```python
from build123d import *

# Parameters (mm, degrees)
SKETCH_1_W                = 80
SKETCH_1_H                = 51
EXTRUDE_1_DEPTH           = 100
SKETCH_2_W                = 30
SKETCH_2_H                = 35
CUT_EXTRUDE_1_DEPTH       = 131.576605868
SKETCH_3_W                = 54
SKETCH_3_H                = 35
CUT_EXTRUDE_2_DEPTH       = 131.576605868
HOLE_WIZARD_1_D           = 9
HOLE_WIZARD_1_CBORE_D     = 15
HOLE_WIZARD_1_CBORE_DEPTH = 9
MM_1_D                    = 6


with BuildPart() as part:
    # 草图1 → 凸台-拉伸1 (new body)
    with BuildSketch(Plane.XY):
        Rectangle(SKETCH_1_W, SKETCH_1_H)
    extrude(amount=EXTRUDE_1_DEPTH)

    # 草图2 → 切除-拉伸1 (cut, through all)
    with BuildSketch(Plane(origin=(40, 0, 0), x_dir=(0, 0, -1), z_dir=(1, 0, 0))):
        with Locations((-85, -8)):
            Rectangle(SKETCH_2_W, SKETCH_2_H)
    extrude(amount=-CUT_EXTRUDE_1_DEPTH, mode=Mode.SUBTRACT)

    # 草图3 → 切除-拉伸2 (cut, through all)
    with BuildSketch(Plane(origin=(40, 0, 0), x_dir=(0, 0, -1), z_dir=(1, 0, 0))):
        with Locations((-27, 8)):
            Rectangle(SKETCH_3_W, SKETCH_3_H)
    extrude(amount=-CUT_EXTRUDE_2_DEPTH, mode=Mode.SUBTRACT)

    # 打孔尺寸(%根据)内六角圆柱头螺钉的类型1 (through all)
    with Locations(Plane(origin=(0, -9.5, 0), x_dir=(1, 0, 0), z_dir=(0, 1, 0))):
        with Locations((-30, -10), (30, -40)):
            CounterBoreHole(HOLE_WIZARD_1_D / 2, HOLE_WIZARD_1_CBORE_D / 2, HOLE_WIZARD_1_CBORE_DEPTH)

    # 大小mm 暗销孔1 (through all)
    with Locations(Plane(origin=(0, -9.5, 0), x_dir=(1, 0, 0), z_dir=(0, 1, 0))):
        with Locations((-30, -40), (30, -10)):
            Hole(MM_1_D / 2)


solid = part.part
```
Model file for the job. Use its own axes, mm. A direction names the side the tool comes from. Coordinates: 2 decimals unless noted, no trailing zeros. Order: outer loops, then holes, each group sorted by start corner. A loop starts at its lowest first (then second) coordinate and runs counter-clockwise, first axis right, second up. Notation, with made-up numbers: (27, -5.5) - (75, -5.5) arc R16 cw to (75, 24.5) - close; hole circle Ø11 at (47.5, 86). An arc over 180 degrees is marked (long way). Return JSON: item names as keys, results as strings. Group by question number.
1) Flat gauge pins, fed straight in: P1, Ø17.5, axis at x = -17, y = -5, coming from the +Z side; P2, Ø16, axis at x = -18, z = 31, coming from the +Y side; P3, Ø7.5, axis at x = 33.5, z = 39, coming from the +Y side. Where does each tip first touch, or does it go through?
2) Saw through at B-B, the plane z = 40. Write the cut outline in (x, y), plus the area to 3 significant figures.
3) Saw through at C-C, the plane y = -13.5. Write the cut outline in (x, z).
4) Mould opens along X. For faces 6 (the cylindrical face through (-34.292, -22.049, 8.648)), 7 (the flat face through (1, 8, 54)), 8 (the flat face through (-40, -12, 49)), 9 (the cylindrical face through (-27.79, -17.61, 37.97)) say: released by +X, released by -X, zero draft, split by the parting line, or undercut.
5) Saw through at A-A, the plane x = -30. Write the cut outline in (y, z), plus the area to 3 significant figures.
6) Tool access for faces 1 (the cylindrical face through (33, -18, 10)), 2 (the flat face through (-1, -17, 0)), 3 (the flat face through (1, -8, 70)), 4 (the flat face through (1, -9.5, 27)), 5 (the cylindrical face through (-37.493, -13.937, 9.67)): list every direction of +Z, -Z, +X, -X, +Y, -Y with a clear straight run to the whole face (end or side of a thin tool).
7) Probe line 1 (Z direction, x = 30, y = -24); line 2 (Z direction, x = -30, y = -23); line 3 (X direction, y = -11.5, z = 40). List the from-to ranges inside material, lowest first. Write a range as from..to.
8) Saw through at D-D, the plane x = 20.5. Write the cut outline in (y, z).
Values found:
{
 "1": {"P1": "stops at z = 70", "P2": "stops at y = -9.5", "P3": "stops at y = -18.5"},
 "2": {"outline": "(-40, -25.5) - (-33, -25.5) - (-33, -9.5) - (-40, -9.5) - close; (-27, -25.5) - (25.5, -25.5) - (25.5, -18.5) - (22.5, -18.5) - (22.5, -9.5) - (-27, -9.5) - close; (34.5, -25.5) - (40, -25.5) - (40, -9.5) - (37.5, -9.5) - (37.5, -18.5) - (34.5, -18.5) - close", "area": "986 mm²"},
 "3": {"outline": "(-40, 0) - (40, 0) - (40, 70) - (-40, 70) - close; hole circle Ø15 at (-30, 10); hole circle Ø6 at (-30, 40); hole circle Ø15 at (30, 40); hole circle Ø6 at (30, 10)"},
 "4": {"face 6": "undercut", "face 7": "zero draft", "face 8": "released by -X", "face 9": "undercut"},
 "5": {"outline": "(-25.5, 0) - (-9.5, 0) - (-9.5, 2.5) - (-18.5, 2.5) - (-18.5, 5.5) - (-25.5, 5.5) - close; (-25.5, 14.5) - (-18.5, 14.5) - (-18.5, 17.5) - (-9.5, 17.5) - (-9.5, 37) - (-25.5, 37) - close; (-25.5, 43) - (-9.5, 43) - (-9.5, 54) - (25.5, 54) - (25.5, 100) - (9.5, 100) - (9.5, 70) - (-25.5, 70) - close", "area": "1,870 mm²"},
 "6": {"face 1": "+Y, -Y", "face 2": "-Z, +X, -X, +Y, -Y", "face 3": "+Z, +X, -X, -Y", "face 4": "-Z, +X, -X, +Y", "face 5": "+Y"},
 "7": {"line 1": "z = 0..7, 13..35.5, 44.5..70", "line 2": "z = 0..5.5, 14.5..37, 43..70", "line 3": "x = -40..-33, -27..22.5, 37.5..40"},
 "8": {"outline": "(-25.5, 0) - (-9.5, 0) - (-9.5, 54) - (25.5, 54) - (25.5, 100) - (9.5, 100) - (9.5, 70) - (-25.5, 70) - close"}
}
